The listing builds one solid part. Answer for the finished solid, in the listing's coordinates (mm). A direction names the side the tool comes from. Coordinates: 2 decimals unless noted, no trailing zeros. Write each loop counter-clockwise with the first axis right and the second up, starting at its lowest first coordinate (ties: lowest second). Pieces come first, ordered by that corner, then holes.
(1) The part is cut by section D-D on y = 21. Determine the outline of the cut face in (x, z) (3 decimals), plus the area to 3 significant figures.
(2) The part is cut by section C-C on z = 8. Determine the outline of the cut face in (x, y), plus the area to 3 significant figures.
(3) Which of the six approach directions +Z, -Z, +X, -X, +Y, -Y give full straight-line access (tool end or side, diameter ignored) to faces 1 (the cylindrical face through (-34.001, -21.391, 4.138)), 2 (the cylindrical face through (34.001, -46.391, 4.138)), 3 (the cylindrical face through (-30.72, 45.49, 4.83))?
(4) The part is cut by section A-A on x = 0. Determine the outline of the cut face in (y, z) (3 decimals).
(5) Given P1, Ø9, axis at x = -10, y = -5, coming from the +Z side (3 decimals); P2, Ø2, axis at x = -27.5, z = 4, coming from the +Y side; P3, Ø2, axis at y = -20, z = 5.025, coming from the -X side; P4, Ø3, axis at y = -20, z = 5.025, coming from the -X side, each flat-ended and moving along its own axis, determine where each tip first touches the part or whether it passes through.
(6) Straight lines are drawn through the part: line 1 (X direction, y = 29, z = 2.25); line 2 (X direction, y = -5, z = 4.5); line 3 (Z direction, x = 34.4, y = -45) (3 decimals). For each, find the intervals that lie inside material, in ascending order.
(7) For a pull along Z with two mould halves and no side action, classify faces 4 (the cylindrical face through (-12.54, -6.05, 4.68)), 5 (the flat face through (0, 1, 0)), 6 (the conical face through (32.181, -20.086, 4.752)) as +Z half, -Z half, draft (parallel to the pull), parting line (faces both ways), or undercut.
(8) The part is cut by section B-B on y = -5. Determine the outline of the cut face in (x, z) (3 decimals), plus the area to 3 significant figures.
from build123d import *

# Parameters (mm, degrees)
SKETCH1_W                             = 70
SKETCH1_H                             = 100
BOSS_EXTRUDE1_DEPTH                   = 9.525
TAP_DRILL_FOR_M4X0_7_TAP1_D           = 3.3
TAP_DRILL_FOR_M4X0_7_TAP1_DEPTH       = 2
TAP_DRILL_FOR_M4X0_7_TAP1_CSINK_D     = 3.35
TAP_DRILL_FOR_M4X0_7_TAP1_CSINK_ANGLE = 90
TAP_DRILL_FOR_M4X0_7_TAP1_TIP         = 0.991420021
SKETCH6_R                             = 7.5
CUT_EXTRUDE1_DEPTH                    = 62.771560001
M5_CLEARANCE_HOLE1_D                  = 5.5
M5_CLEARANCE_HOLE1_CSINK_D            = 5.55
M5_CLEARANCE_HOLE1_CSINK_ANGLE        = 90
TAP_DRILL_FOR_M4X0_7_TAP2_AT_2_COUNT  = 2
TAP_DRILL_FOR_M4X0_7_TAP2_AT_2_PITCH  = 25
FILLET1_R                             = 15


with BuildPart() as part:
    # Sketch1 → Boss-Extrude1 (new body)
    with BuildSketch(Plane.XY):
        Rectangle(SKETCH1_W, SKETCH1_H)
    extrude(amount=BOSS_EXTRUDE1_DEPTH)

    # Tap Drill for M4x0.7 Tap1
    with Locations(Plane(origin=(0, -50, 0), x_dir=(-1, 0, 0), z_dir=(0, -1, 0))):
        with Locations((20, -4.7625), (-20, -4.7625)):
            CounterSinkHole(TAP_DRILL_FOR_M4X0_7_TAP1_D / 2, TAP_DRILL_FOR_M4X0_7_TAP1_CSINK_D / 2, depth=TAP_DRILL_FOR_M4X0_7_TAP1_DEPTH, counter_sink_angle=TAP_DRILL_FOR_M4X0_7_TAP1_CSINK_ANGLE)
            with Locations((0, 0, -(TAP_DRILL_FOR_M4X0_7_TAP1_DEPTH + TAP_DRILL_FOR_M4X0_7_TAP1_TIP / 2))):  # 118° drill point
                Cone(0, TAP_DRILL_FOR_M4X0_7_TAP1_D / 2, TAP_DRILL_FOR_M4X0_7_TAP1_TIP, mode=Mode.SUBTRACT)

    # Sketch6 → Cut-Extrude1 (cut, through all)
    with BuildSketch(Plane.XY.offset(9.525)):
        with Locations((0, 21)):
            Circle(SKETCH6_R)
    extrude(amount=-CUT_EXTRUDE1_DEPTH, mode=Mode.SUBTRACT)

    # M5 Clearance Hole1 (through all)
    with Locations(Plane.XY.offset(9.525)):
        with Locations((-10, -5), (10, -5), (24, 9), (24, 29), (-24, 9), (-24, 29)):
            CounterSinkHole(M5_CLEARANCE_HOLE1_D / 2, M5_CLEARANCE_HOLE1_CSINK_D / 2, counter_sink_angle=M5_CLEARANCE_HOLE1_CSINK_ANGLE)

    # Sketch16 → Tap Drill for M4x0.7 Tap2 (revolve, cut)
    with BuildSketch(Plane(origin=(35, -45, 5.025), x_dir=(0, 0, -1), z_dir=(0, 1, 0))):
        Polygon((0, 0), (0, 2.991420021), (1.65, 2), (1.65, 0.025), (1.675, 0), align=None)
    tap_drill_for_m4x0_7_tap2 = revolve(axis=Axis((41.35, -45, 5.025), (-1, 0, 0)), mode=Mode.SUBTRACT)

    # Tap Drill for M4x0.7 Tap2 at 2: Tap Drill for M4x0.7 Tap2 ×2
    with Locations(*[(0, i * TAP_DRILL_FOR_M4X0_7_TAP2_AT_2_PITCH, 0) for i in range(1, TAP_DRILL_FOR_M4X0_7_TAP2_AT_2_COUNT)]):
        add(tap_drill_for_m4x0_7_tap2, mode=Mode.SUBTRACT)

    # Mirror1: Tap Drill for M4x0.7 Tap2 across plane
    add(tap_drill_for_m4x0_7_tap2.mirror(Plane(origin=(0, 0, 0), x_dir=(0, 0, 1), z_dir=(1, 0, 0))), mode=Mode.SUBTRACT)

    # Mirror1 copy 1 sketch → Mirror1 copy 1 (revolve, cut)
    with BuildSketch(Plane(origin=(-35, -20, 5.025), x_dir=(0, 0, -1), z_dir=(0, 1, 0))):
        Polygon((0, 0), (0, -2.991420021), (1.65, -2), (1.65, -0.025), (1.675, 0), align=None)
    revolve(axis=Axis((-41.35, -20, 5.025), (-1, 0, 0)), mode=Mode.SUBTRACT)

    # Fillet1
    fillet1_edges = [part.edges().sort_by_distance(p)[0] for p in [
        (-35, 50, 4.7625),
        (35, 50, 4.7625),
    ]]
    fillet(fillet1_edges, radius=FILLET1_R)


solid = part.part
Model answer:
1. outline: (-35, 0) - (-7.5, 0) - (-7.5, 9.525) - (-35, 9.525) - close; (7.5, 0) - (35, 0) - (35, 9.525) - (7.5, 9.525) - close
1. area: 524 mm2
2. outline: (-35, -50) - (35, -50) - (35, 35) arc R15 ccw to (20, 50) - (-20, 50) arc R15 ccw to (-35, 35) - close; hole circle Ø5.5 at (-24, 9); hole circle Ø5.5 at (-24, 29); hole circle Ø5.5 at (-10, -5); hole circle Ø15 at (0, 21); hole circle Ø5.5 at (10, -5); hole circle Ø5.5 at (24, 9); hole circle Ø5.5 at (24, 29)
2. area: 6,580 mm2
3. face 1: -X
3. face 2: +X
3. face 3: +Z, -Z, -X, +Y
4. outline: (-50, 0) - (13.5, 0) - (13.5, 9.525) - (-50, 9.525) - close; (28.5, 0) - (50, 0) - (50, 9.525) - (28.5, 9.525) - close
5. P1: stops at z = 9.525
5. P2: stops at y = 48.52
5. P3: stops at x = -32.61
5. P4: stops at x = -32.91
6. line 1: x = -35 to -26.75, -21.25 to 21.25, 26.75 to 35
6. line 2: x = -35 to -12.75, -7.25 to 7.25, 12.75 to 35
6. line 3: z = 0 to 3.375, 6.675 to 9.525
7. face 4: draft
7. face 5: -Z half
7. face 6: undercut
8. outline: (-35, 0) - (-12.75, 0) - (-12.75, 9.5) - (-12.775, 9.525) - (-35, 9.525) - close; (-7.25, 0) - (7.25, 0) - (7.25, 9.5) - (7.225, 9.525) - (-7.225, 9.525) - (-7.25, 9.5) - close; (12.75, 0) - (35, 0) - (35, 9.525) - (12.775, 9.525) - (12.75, 9.5) - close
8. area: 562 mm2
